```python
from build123d import *

# Parameters (mm, degrees)
SKETCH_1_R      = 27.5
EXTRUDE_1_DEPTH = 6
EXTRUDE_1_TAPER = -16
EXTRUDE_2_DEPTH = 2


with BuildPart() as part:
    # Эскиз1 → Бобышка-Вытянуть1 (new body)
    with BuildSketch(Plane.XY):
        with Locations((0, 27.755280905)):
            Circle(SKETCH_1_R)
    extrude(amount=EXTRUDE_1_DEPTH, taper=EXTRUDE_1_TAPER)

    # Эскиз3 → Бобышка-Вытянуть2 (add)
    with BuildSketch(Plane.XY.offset(6)):
        with BuildLine():
            Line((-32, 78.755280905), (32, 78.755280905))
            ThreePointArc((32, 78.755280905), (39.071067812, 75.826348716), (42, 68.755280905))
            Line((42, 68.755280905), (42, -13.244719095))
            ThreePointArc((42, -13.244719095), (39.071067812, -20.315786907), (32, -23.244719095))
            Line((32, -23.244719095), (-32, -23.244719095))
            ThreePointArc((-32, -23.244719095), (-39.071067812, -20.315786907), (-42, -13.244719095))
            Line((-42, -13.244719095), (-42, 68.755280905))
            ThreePointArc((-42, 68.755280905), (-39.071067812, 75.826348716), (-32, 78.755280905))
        make_face()
        with BuildLine():
            Line((-29.900944715, 71.142300912), (-26.722408451, 67.282649734))
            ThreePointArc((-26.722408451, 67.282649734), (-27.335411873, 60.948281036), (-33.669780571, 61.561284458))
            Line((-33.669780571, 61.561284458), (-36.848316835, 65.420935637))
            ThreePointArc((-36.848316835, 65.420935637), (-36.235313413, 71.755304335), (-29.900944715, 71.142300912))
        make_face(mode=Mode.SUBTRACT)
        with BuildLine():
            Line((36.848316835, 65.420935637), (33.669780571, 61.561284458))
            ThreePointArc((33.669780571, 61.561284458), (27.335411873, 60.948281036), (26.722408451, 67.282649734))
            Line((26.722408451, 67.282649734), (29.900944715, 71.142300912))
            ThreePointArc((29.900944715, 71.142300912), (36.235313413, 71.755304335), (36.848316835, 65.420935637))
        make_face(mode=Mode.SUBTRACT)
        with BuildLine():
            Line((29.900944715, -15.631739103), (26.722408451, -11.772087925))
            ThreePointArc((26.722408451, -11.772087925), (27.335411873, -5.437719227), (33.669780571, -6.050722649))
            Line((33.669780571, -6.050722649), (36.848316835, -9.910373827))
            ThreePointArc((36.848316835, -9.910373827), (36.235313413, -16.244742526), (29.900944715, -15.631739103))
        make_face(mode=Mode.SUBTRACT)
        with BuildLine():
            Line((-36.848316835, -9.910373827), (-33.669780571, -6.050722649))
            ThreePointArc((-33.669780571, -6.050722649), (-27.335411873, -5.437719227), (-26.722408451, -11.772087925))
            Line((-26.722408451, -11.772087925), (-29.900944715, -15.631739103))
            ThreePointArc((-29.900944715, -15.631739103), (-36.235313413, -16.244742526), (-36.848316835, -9.910373827))
        make_face(mode=Mode.SUBTRACT)
    extrude(amount=EXTRUDE_2_DEPTH)


solid = part.part
```
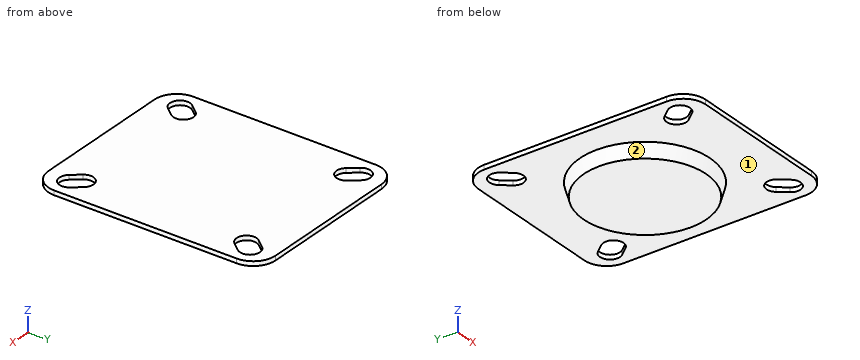
Work out the finished part from the listing and answer in its coordinate system (mm). Face numbers are marked on the shaded views. Coordinates: 2 decimals unless noted, no trailing zeros. Loops run counter-clockwise (first coordinate to the right, second up) from the corner with the lowest first, then second, coordinate; pieces in that order, holes last. Notation, with made-up numbers: M -9.75,34.5 L 17.25,34.5 A19 ccw 17.25,42.5 Z; hole C 20,32 d4. An arc over 180 degrees is marked long. Use CSV: the item, a comma, the result in double quotes. Start each with the question number.
(1) Given pin 1 Ø1 at (x, z) = (15.5, 4.5) entering from +Y; pin 2 Ø1 at (x, z) = (22, 2.5) entering from -Y; pin 3 Ø6 at (x, y) = (-21.5, -5) entering from -Z, each flat-ended and moving along its own axis, determine where each tip first touches the part or whether it passes through.
(2) Find section B-B, the plane z = 1.75. Give the vertices of the cut face in (x, y).
(3) Find section A-A, the plane x = 0. Give the vertices of the cut face in (y, z).
(4) For a pull along X with two mould halves and no side action, classify the marked faces 1 and 2 as +X half, -X half, draft (parallel to the pull), parting line (faces both ways), or undercut.
(5) Consider line 1 (Y direction, x = 31, z = 6.5); line 2 (X direction, y = 71, z = 7.75); line 3 (Y direction, x = -27, z = 6.75). Determine where each line is inside the solid, lowest interval first.
Recorded:
1,pin 1,"stops at y = 52.37"
1,pin 2,"stops at y = 9.44"
1,pin 3,"stops at z = 6"
2,outline,"C 0,27.76 d56"
3,outline,"M -23.24,6 L -1.47,6 L 0.26,0 L 55.26,0 L 56.98,6 L 78.76,6 L 78.76,8 L -23.24,8 Z"
4,face 1,"draft"
4,face 2,"parting line"
5,line 1,"y = -23.24 to -16.59, -4.48 to 59.99, 72.1 to 78.76"
5,line 2,"x = -41.74 to -36.96, -29.78 to 29.78, 36.96 to 41.74"
5,line 3,"y = -23.24 to -12.11, -5.74 to 61.25, 67.62 to 78.76"
